The listing builds one solid part. Answer for the finished solid, in the listing's coordinates (mm). A direction names the side the tool comes from. Round coordinates to 2 decimals unless told otherwise and drop trailing zeros. Order: outer loops, then holes, each group sorted by start corner. A loop starts at its lowest first (then second) coordinate and runs counter-clockwise, first axis right, second up. Notation, with made-up numbers: M -21.75,55 L 35.25,55 A10 cw 35.25,67 Z; hole C -12.5,68 d1. An arc over 180 degrees is marked long. Put each result on its own line as item: value. Start each with the question number.
1. The part is cut by section B-B (z = 26.5). Give the vertices of the cut face in (x, y).
2. The part is cut by section A-A (z = 72). Give the vertices of the cut face in (x, y), then the cut area to 3 significant figures.
3. The part is cut by section D-D (x = 6.5). Give the vertices of the cut face in (y, z), then the cut area to 3 significant figures.
4. The part is cut by section C-C (y = 11.25). Give the vertices of the cut face in (x, z).
5. Consider line 1 (Z direction, x = 14.5, y = 7); line 2 (Y direction, x = 12.5, z = 146); line 3 (X direction, y = 13.5, z = 37). Determine where each line is inside the solid, lowest interval first.
6. Which of the six approach directions +Z, -Z, +X, -X, +Y, -Y give full straight-line access (tool end or side, diameter ignored) to faces 1 (the face through (9, 9, 99)), 2 (the face through (9, 6, 99)), 3 (the face through (21.45, 7.52, 148.7))?
7. Each of these flat-tipped pins is pushed along its axis until it touches: pin 1 Ø2.5 at (x, y) = (14, 8) entering from -Z; pin 2 Ø8 at (x, y) = (18.5, 8) entering from +Z; pin 3 Ø6.5 at (x, z) = (9.5, 84) entering from +Y. Where does it stop, or does it pass through?
from build123d import *

# Parameters (mm, degrees)
SKETCH_1_W          = 3
SKETCH_1_H          = 15
EXTRUDE_1_DEPTH     = 200
EXTRUDE_7_DEPTH     = 3
SKETCH_13_W         = 3.3
SKETCH_13_H         = 10.3
SKETCH_13_W_2       = 8.9
SKETCH_13_H_2       = 4.4
CUT_EXTRUDE_1_DEPTH = 10


with BuildPart() as part:
    # 草图1 → 凸台-拉伸1 (new body)
    with BuildSketch(Plane.XY):
        with Locations((1.5, 7.5)):
            Rectangle(SKETCH_1_W, SKETCH_1_H)
    extrude(amount=EXTRUDE_1_DEPTH)

    # 草图12 → 凸台-拉伸7 (add)
    with BuildSketch(Plane(origin=(0, 9, 0), x_dir=(1, 0, 0), z_dir=(0, 1, 0))):
        Polygon((18, -191.190016229), (25, -105), (25, -95), (18, -8.809983771), (3, -8.809983771), (3, -191.190016229), align=None)
    extrude(amount=-EXTRUDE_7_DEPTH)

    # 草图13 → 切除-拉伸1 (cut)
    with BuildSketch(Plane.XZ.offset(-6)):
        with Locations((12.5, 29.999983771)):
            Rectangle(SKETCH_13_W, SKETCH_13_H)
        with Locations((12.5, 169.999983771)):
            Rectangle(SKETCH_13_W, SKETCH_13_H)
        with Locations((15.25, 99.999983771)):
            Rectangle(SKETCH_13_W_2, SKETCH_13_H_2)
    extrude(amount=-CUT_EXTRUDE_1_DEPTH, mode=Mode.SUBTRACT)


solid = part.part
Resolved:
1. outline: M 0,0 L 3,0 L 3,6 L 10.85,6 L 10.85,9 L 3,9 L 3,15 L 0,15 Z; M 14.15,6 L 19.44,6 L 19.44,9 L 14.15,9 Z
2. outline: M 0,0 L 3,0 L 3,6 L 23.13,6 L 23.13,9 L 3,9 L 3,15 L 0,15 Z
2. area: 105 mm2
3. outline: M 6,8.81 L 9,8.81 L 9,191.19 L 6,191.19 Z
3. area: 547 mm2
4. outline: M 0,0 L 3,0 L 3,200 L 0,200 Z
5. line 1: 8.81 to 97.8, 102.2 to 191.19
5. line 2: 6 to 9
5. line 3: 0 to 3
6. face 1: +Z, -Z, +X, +Y
6. face 2: +Z, -Z, +X, -Y
6. face 3: +Z, +X, +Y, -Y
7. pin 1: z = 8.81
7. pin 2: z = 191.19
7. pin 3: y = 9
